Verification items for the finished model (mm, model axes). Face numbers are marked on the shaded views. A direction names the side the tool comes from. Coordinates: 2 decimals unless noted, no trailing zeros. Write each loop counter-clockwise with the first axis right and the second up, starting at its lowest first coordinate (ties: lowest second). Pieces come first, ordered by that corner, then holes. Notation, with made-up numbers: (84, -38.75) - (103, -38.75) arc R24 cw to (103, -13.75) - close; hole circle Ø11 at (-7, -15). An arc over 180 degrees is marked (long way). Answer as CSV lines item,"result". Start each with the question number.
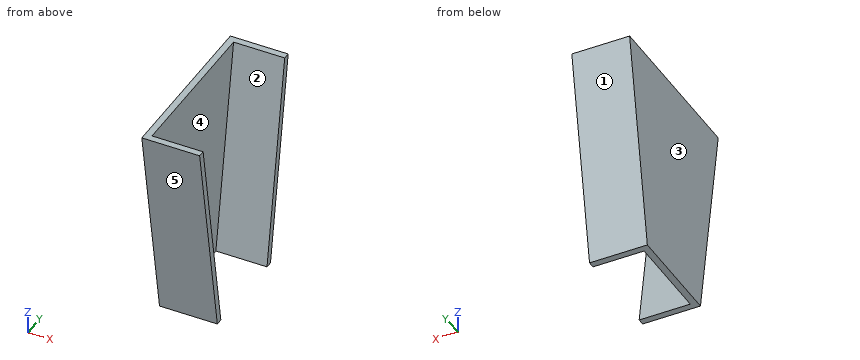
Autodesk Inventor part; units mm, degrees
ref_plane "YZ Plane" through (0, 0, 0) normal (1, 0, 0) x (0, 1, 0)
ref_plane "XZ Plane" through (0, 0, 0) normal (0, 1, 0) x (-1, 0, 0)
ref_plane "XY Plane" through (0, 0, 0) normal (0, 0, 1) x (1, 0, 0)
sketch "Sketch3" plane through (0, 0, 0) normal (1, 0, 0) x (0, 1, 0)
  line L0 (0, 155.5521) -> (-254, 155.5521)
  line L1 (-254, 155.5521) -> (-254, 0)
  line L2 (-254, 0) -> (0, 0)
  line L3 (0, 0) -> (0, 155.5521)
  dimension "d0" = 254
extrude "Extrusion1" add sketch "Sketch3" along normal blind 5
sketch "Sketch4" plane through (0, 0, 0) normal (-1, 0, 0) x (0, 0, 1)
  line L0 (155.5521, 0) -> (155.5521, -254) construction
  line L1 (0, 0) -> (155.5521, 0)
  line L2 (0, -254) -> (0, 0) construction
  line L3 (155.5521, -254) -> (0, -254)
  line L4 (0, 0) -> (0, -88.9)
  line L5 (0, -254) -> (0, 0)
  line L6 (155.5521, 0) -> (0, 0)
  line L7 (155.5521, -254) -> (0, -254)
  line L8 (0, -254) -> (0, -165.1)
  line L9 (155.5521, -254) -> (155.5521, -190.5)
  line L10 (155.5521, 0) -> (155.5521, -254)
  line L11 (155.5521, -190.5) -> (0, -165.1)
  line L12 (155.5521, 0) -> (155.5521, -63.5)
  line L13 (155.5521, -63.5) -> (0, -88.9)
  dimension "d3" = 88.9
  dimension "d4" = 88.9
  dimension "d5" = 63.5
  dimension "d7" = 63.5
  dimension "d10" = 155.5521
extrude "Extrusion2" cut sketch "Sketch4" against normal through all contours L1 L10 L13 L4 | L11 L9 L3 L5
sketch "Sketch7" plane through (5, 0, 0) normal (1, 0, 0) x (0, 0, -1)
  line L0 (-155.5521, -190.5) -> (0, -165.1)
  line L1 (0, -165.1) -> (0, -88.9)
  line L2 (0, -88.9) -> (-155.5521, -63.5)
  line L3 (-155.5521, -63.5) -> (-155.5521, -190.5)
  line L4 (0, -88.9) -> (-155.5521, -63.5)
  line L5 (-155.5521, -63.5) -> (-155.5521, -68.5)
  line L6 (-155.5521, -63.5) -> (-155.5521, -190.5)
  line L7 (0, -88.9) -> (0, -93.9)
  line L8 (0, -165.1) -> (0, -88.9)
  line L9 (0, -93.9) -> (-155.5521, -68.5)
  line L10 (-155.5521, -190.5) -> (-155.5521, -185.5)
  line L11 (-155.5521, -185.5) -> (0, -160.1)
  line L12 (0, -165.1) -> (-154.7568, -190.3701)
  line L13 (0, -165.1) -> (-155.5521, -190.5)
  point P0 (0, 0)
  dimension "d14" = 5
  dimension "d15" = 5
extrude "Extrusion3" add sketch "Sketch7" along normal blind 38.1 contours L3 L11 L1 L0 | L3 L2 L1 L9
1. Access from +Z, -Z, +X, -X, +Y, -Y to the whole of each face (thin tool, end or side, straight path). Record for the marked faces 4 and 5.
2. Scan lines: line 1 along X through (y, z) = (-153, 14); line 2 along Y through (x, z) = (27.5, 143); line 3 along Y through (x, z) = (7, 107.5). Record each from-to range of solid material in increasing order. Write a range as from..to.
3. Cross-section at B-B (z = 71). Record the cut outline in (x, y), and give its area (3 significant figures).
4. Cross-section at D-D (z = 52.5). Record the cut outline in (x, y).
5. Cross-section at A-A (x = 35.5). Record the cut outline in (y, z).
6. Cross-section at C-C (y = -125.5). Record the cut outline in (x, z).
7. Draft check along Y on the marked faces 1, 2 and 3. Enter one of: pulls with the +Y half, pulls with the -Y half, needs draft (parallel to the pull), parting line crosses it, or undercut.
8. Depth check by flat-ended pin: P1, Ø6, axis at x = 31.5, z = 113, coming from the +Y side; P2, Ø1.5, axis at y = -82.5, z = 130, coming from the +X side; P3, Ø10, axis at x = 35.5, z = 76.5, coming from the +Y side; P4, Ø3, axis at y = -78, z = 54.5, coming from the +X side. Enter the tip coordinate at first touch or a pass-through.
Completed:
1,face 4,"+Z, +X"
1,face 5,"-Z, +X, -X, -Y"
2,line 1,"x = 0..5"
2,line 2,"y = -188.45..-183.45, -70.55..-65.55"
2,line 3,"y = -182.65..-177.65, -76.35..-71.35"
3,outline,"(0, -176.69) - (43.1, -176.69) - (43.1, -171.69) - (5, -171.69) - (5, -82.31) - (43.1, -82.31) - (43.1, -77.31) - (0, -77.31) - close"
3,area,"878 mm2"
4,outline,"(0, -173.67) - (43.1, -173.67) - (43.1, -168.67) - (5, -168.67) - (5, -85.33) - (43.1, -85.33) - (43.1, -80.33) - (0, -80.33) - close"
5,outline,"(-190.5, 155.55) - (-165.1, 0) - (-160.1, 0) - (-185.5, 155.55) - close; (-93.9, 0) - (-88.9, 0) - (-63.5, 155.55) - (-68.5, 155.55) - close"
6,outline,"(0, 0) - (5, 0) - (5, 155.55) - (0, 155.55) - close"
7,face 1,"pulls with the +Y half"
7,face 2,"undercut"
7,face 3,"needs draft"
8,P1,"stops at y = -69.96"
8,P2,"stops at x = 5"
8,P3,"stops at y = -75.59"
8,P4,"passes through"
